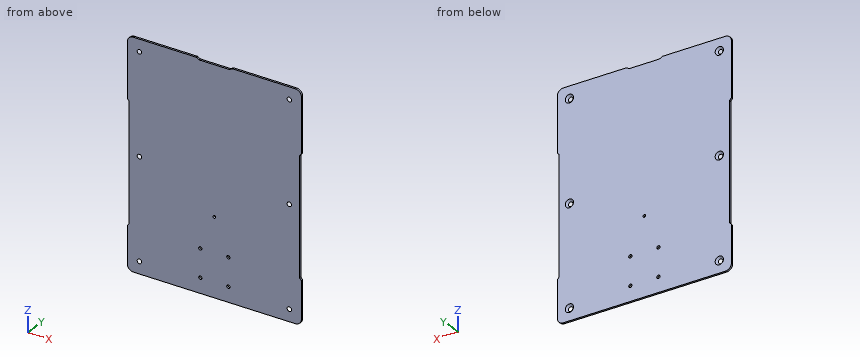
from build123d import *

# Parameters (mm, degrees)
SKETCH1_W           = 360
SKETCH1_H           = 464
SKETCH1_R           = 3.4
SKETCH1_R_2         = 2.731026391
BOSS_EXTRUDE1_DEPTH = 4
FILLET1_R           = 12.5
SKETCH5_R           = 3.4
CUT_EXTRUDE4_DEPTH  = 20
CUT_EXTRUDE5_DEPTH  = 10
CUT_EXTRUDE6_DEPTH  = 10
FILLET2_R           = 3
CHAMFER1_SIZE       = 5.15


with BuildPart() as part:
    # Sketch1 → Boss-Extrude1 (new body)
    with BuildSketch(Plane(origin=(0, 30, 0), x_dir=(1, 0, 0), z_dir=(0, 1, 0))):
        Rectangle(SKETCH1_W, SKETCH1_H)
        with Locations(Location((-155, 207, 0), (0, 0, 270))):
            Circle(SKETCH1_R, mode=Mode.SUBTRACT)
        with Locations(Location((155, 207, 0), (0, 0, 90))):
            Circle(SKETCH1_R, mode=Mode.SUBTRACT)
        with Locations(Location((-155, -207, 0), (0, 0, 270))):
            Circle(SKETCH1_R, mode=Mode.SUBTRACT)
        with Locations(Location((155, -207, 0), (0, 0, 90))):
            Circle(SKETCH1_R, mode=Mode.SUBTRACT)
        with Locations(Location((-155, 0, 0), (0, 0, 270))):
            Circle(SKETCH1_R, mode=Mode.SUBTRACT)
        with Locations(Location((155, 0, 0), (0, 0, 90))):
            Circle(SKETCH1_R, mode=Mode.SUBTRACT)
        with Locations(Location((0, 72, 0), (0, 0, 270))):
            Circle(SKETCH1_R_2, mode=Mode.SUBTRACT)
    extrude(amount=-BOSS_EXTRUDE1_DEPTH)

    # Fillet1
    fillet1_edges = [part.edges().sort_by_distance(p)[0] for p in [
        (180, 28, -232),
        (180, 28, 232),
        (-180, 28, 232),
        (-180, 28, -232),
    ]]
    fillet(fillet1_edges, radius=FILLET1_R)

    # Sketch5 → Cut-Extrude4 (cut)
    with BuildSketch(Plane(origin=(0, 40, 377.333920735), x_dir=(0, 0, 1), z_dir=(0, 1, 0))):
        with Locations((-520.342542706, 28.991378029)):
            Circle(SKETCH5_R)
        with Locations((-520.342542706, -28.991378029)):
            Circle(SKETCH5_R)
        with Locations((-578.325298763, -28.991378029)):
            Circle(SKETCH5_R)
        with Locations((-578.325298763, 28.991378029)):
            Circle(SKETCH5_R)
    extrude(amount=-CUT_EXTRUDE4_DEPTH, mode=Mode.SUBTRACT)

    # Sketch6 → Cut-Extrude5 (cut)
    with BuildSketch(Plane(origin=(0, 30, 0), x_dir=(1, 0, 0), z_dir=(0, 1, 0))):
        Polygon((-176, -102.929588377), (-176, 139.070411623), (-188.727922061, 151.798333685), (-188.727922061, -115.657510438), align=None)
    cut_extrude5 = extrude(amount=-CUT_EXTRUDE5_DEPTH, mode=Mode.SUBTRACT)

    # Sketch7 → Cut-Extrude6 (cut)
    with BuildSketch(Plane(origin=(0, 30, 0), x_dir=(1, 0, 0), z_dir=(0, 1, 0))):
        Polygon((-31.320564901, -228.594250629), (31.320564901, -228.594250629), (45, -236.893229805), (-45, -236.893229805), align=None)
    extrude(amount=-CUT_EXTRUDE6_DEPTH, mode=Mode.SUBTRACT)

    # Mirror2: Cut-Extrude5 across plane
    add(cut_extrude5.mirror(Plane(origin=(0, 0, 0), x_dir=(0, 0, 1), z_dir=(1, 0, 0))), mode=Mode.SUBTRACT)

    # Fillet2
    fillet2_edges = [part.edges().sort_by_distance(p)[0] for p in [
        (36.934355042, 28, 232),
        (-36.934355042, 28, 232),
        (-31.320564901, 28, 228.594250629),
        (31.320564901, 28, 228.594250629),
        (176, 28, 102.929588377),
        (176, 28, -139.070411623),
        (-176, 28, -139.070411623),
        (-176, 28, 102.929588377),
    ]]
    fillet(fillet2_edges, radius=FILLET2_R)

    # Chamfer1
    # the kernel refuses this chamfer: 5.15 mm, written as the material it takes off along each edge
    with BuildSketch(Plane(origin=(-155, 30, -207), x_dir=(0, 0, 1), z_dir=(-1, 0, 0))) as chamfer1_piece_1:
        Polygon((3.4 + CHAMFER1_SIZE, 0), (3.4, -CHAMFER1_SIZE), (3.4, 0), align=None)
    revolve(axis=Axis((-155, 30, -207), (0, 1, 0)), mode=Mode.SUBTRACT)
    with BuildSketch(Plane(origin=(155, 30, 207), x_dir=(0, 0, -1), z_dir=(1, 0, 0))) as chamfer1_piece_2:
        Polygon((3.4 + CHAMFER1_SIZE, 0), (3.4, -CHAMFER1_SIZE), (3.4, 0), align=None)
    revolve(axis=Axis((155, 30, 207), (0, 1, 0)), mode=Mode.SUBTRACT)
    with BuildSketch(Plane(origin=(155, 30, 0), x_dir=(0, 0, -1), z_dir=(1, 0, 0))) as chamfer1_piece_3:
        Polygon((3.4 + CHAMFER1_SIZE, 0), (3.4, -CHAMFER1_SIZE), (3.4, 0), align=None)
    revolve(axis=Axis((155, 30, 0), (0, 1, 0)), mode=Mode.SUBTRACT)
    with BuildSketch(Plane(origin=(-155, 30, 207), x_dir=(0, 0, 1), z_dir=(-1, 0, 0))) as chamfer1_piece_4:
        Polygon((3.4 + CHAMFER1_SIZE, 0), (3.4, -CHAMFER1_SIZE), (3.4, 0), align=None)
    revolve(axis=Axis((-155, 30, 207), (0, 1, 0)), mode=Mode.SUBTRACT)
    with BuildSketch(Plane(origin=(-155, 30, 0), x_dir=(0, 0, 1), z_dir=(-1, 0, 0))) as chamfer1_piece_5:
        Polygon((3.4 + CHAMFER1_SIZE, 0), (3.4, -CHAMFER1_SIZE), (3.4, 0), align=None)
    revolve(axis=Axis((-155, 30, 0), (0, 1, 0)), mode=Mode.SUBTRACT)
    with BuildSketch(Plane(origin=(155, 30, -207), x_dir=(0, 0, -1), z_dir=(1, 0, 0))) as chamfer1_piece_6:
        Polygon((3.4 + CHAMFER1_SIZE, 0), (3.4, -CHAMFER1_SIZE), (3.4, 0), align=None)
    revolve(axis=Axis((155, 30, -207), (0, 1, 0)), mode=Mode.SUBTRACT)


solid = part.part
Input: part model. Units: mm. Frame: model coordinates. Give positions to 0.01 mm unless a question says otherwise; leave off trailing zeros. Loops run counter-clockwise (first coordinate to the right, second up) from the corner with the lowest first, then second, coordinate; pieces in that order, holes last. Notation, with made-up numbers: M 72.5,14.5 L 112.5,14.5 A16 ccw 112.5,38.5 Z; hole C 30,89.5 d10. An arc over 180 degrees is marked long. Use CSV: the item, a comma, the result in double quotes.
(1) Section A-A, the plane x = 155. Return loops of the section in (y, z), plus the area to 3 significant figures.
Outcome:
outline,"M 26,-232 L 30,-232 L 30,-215.55 L 26,-211.55 Z; M 26,-202.45 L 30,-198.45 L 30,-8.55 L 26,-4.55 Z; M 26,4.55 L 30,8.55 L 30,198.45 L 26,202.45 Z; M 26,211.55 L 30,215.55 L 30,232 L 26,232 Z"
area,"1,700 mm²"
(2) Pin query (flat end, axial travel): P1, Ø1, axis at y = 26.5, z = 24, coming from the +X side; P2, Ø11, axis at x = 28.99, z = -143.01, coming from the -Y side; P3, Ø6, axis at x = -28.99, z = -200.99, coming from the -Y side. Return the tip coordinate at first contact, or that it passes through.
Outcome:
P1,"stops at x = 176"
P2,"stops at y = 26"
P3,"passes through"
(3) Section C-C, the plane y = 28.35. Count the separate pieces of the cut face and the enclosed holes in it, plus the area to 3 significant figures.
Outcome:
separate pieces,"1"
enclosed holes,"11"
area,"164,000 mm²"
(4) Section B-B, the plane z = -85.5. Return loops of the section in (x, y), plus the area to 3 significant figures.
Outcome:
outline,"M -176,26 L 176,26 L 176,30 L -176,30 Z"
area,"1,410 mm²"
(5) Material intervals for L1, parallel to Z at x = -30.5, y = 27.7; L2, parallel to X at y = 27.7, z = 0; L3, parallel to X at y = 28.1, z = -5, sorted ascending. Write a range as [from, to].
Outcome:
L1,"z = [-232, -204.04], [-197.94, -146.06], [-139.96, 228.59]"
L2,"x = [-176, -161.25], [-148.75, 148.75], [161.25, 176]"
L3,"x = [-176, -159.38], [-150.62, 150.62], [159.38, 176]"
